Read the model definition and answer for the solid it produces. Units are mm, in the model's axes. A direction names the side the tool comes from. Coordinates: 2 decimals unless noted, no trailing zeros. Write each loop counter-clockwise with the first axis right and the second up, starting at its lowest first coordinate (ties: lowest second). Pieces come first, ordered by that corner, then holes.
1) The part is cut by section B-B (x = -1). Determine the outline of the cut face in (y, z), then the cut area to 3 significant figures.
2) The part is cut by section A-A (y = 0). Determine the outline of the cut face in (x, z).
3) The part is cut by section C-C (z = -6). Determine the outline of the cut face in (x, y).
4) Which of the six approach directions +Z, -Z, +X, -X, +Y, -Y give full straight-line access (tool end or side, diameter ignored) to faces 4 (the face through (-8, 0, 32.5)), 5 (the face through (8, 2.301, 31)), 6 (the face through (-0.218, 0.976, -9.535)), 7 (the face through (3, 0, -1)), 8 (the face through (-7.001, 0, 30.5))?
5) Each of these flat-tipped pins is pushed along its axis until it touches: pin 1 Ø0.6 at (x, z) = (7.5, 31.5) entering from +Y; pin 2 Ø6 at (x, z) = (3.5, 5) entering from -Y; pin 3 Ø0.6 at (x, z) = (-8, 32) entering from -Y. Where does it stop, or does it pass through?
6) Determine the mould class of faces 1 (the face through (8, 0, 32.5)), 2 (the face through (-0.2, 1.3, -7)), 3 (the face through (8.188, 0, 30.5)) for opening direction Z: +Z half, -Z half, draft (parallel to the pull), parting line (faces both ways), or undercut.
7) The part is cut by section D-D (y = -3.5). Determine the outline of the cut face in (x, z), then the cut area to 3 significant figures.
8) Find the intervals of material crossed by line 1 (Z direction, x = -3, y = -9.25); line 2 (Z direction, x = -2, y = 0.75); line 3 (Y direction, x = 0.5, z = 26), in increasing order.
from build123d import *

# Parameters (mm, degrees)
SKETCH1_R           = 11
BOSS_EXTRUDE1_DEPTH = 30
SKETCH2_R           = 3
BOSS_EXTRUDE2_DEPTH = 2
SKETCH3_R           = 2
BOSS_EXTRUDE3_DEPTH = 10
SKETCH4_W           = 1.187251635
SKETCH4_H           = 4.601713706
BOSS_EXTRUDE4_DEPTH = 3
SKETCH5_W           = 1.771317087
SKETCH5_H           = 3.201713706
CUT_EXTRUDE1_DEPTH  = 40.726440378
CUT_EXTRUDE2_DEPTH  = 5


with BuildPart() as part:
    # Sketch1 → Boss-Extrude1 (new body)
    with BuildSketch(Plane.XY):
        Circle(SKETCH1_R)
    extrude(amount=BOSS_EXTRUDE1_DEPTH)

    # Sketch2 → Boss-Extrude2 (add)
    with BuildSketch(Plane(origin=(0, 0, 0), x_dir=(-1, 0, 0), z_dir=(0, 0, -1))):
        Circle(SKETCH2_R)
    extrude(amount=BOSS_EXTRUDE2_DEPTH)

    # Sketch3 → Boss-Extrude3 (add)
    with BuildSketch(Plane(origin=(0, 0, -2), x_dir=(-1, 0, 0), z_dir=(0, 0, -1))):
        Circle(SKETCH3_R)
    extrude(amount=BOSS_EXTRUDE3_DEPTH)

    # Sketch4 → Boss-Extrude4 (add)
    with BuildSketch(Plane.XY.offset(30)):
        with Locations((-7.594653551, 0)):
            Rectangle(SKETCH4_W, SKETCH4_H)
        with Locations((7.594653551, 0)):
            Rectangle(SKETCH4_W, SKETCH4_H)
    extrude(amount=BOSS_EXTRUDE4_DEPTH)

    # Sketch5 → Cut-Extrude1 (cut, through all)
    with BuildSketch(Plane.ZY.offset(8.188279368)):
        with Locations((31.614341457, 0)):
            Rectangle(SKETCH5_W, SKETCH5_H)
    extrude(amount=-CUT_EXTRUDE1_DEPTH, mode=Mode.SUBTRACT)

    # Sketch6 → Cut-Extrude2 (cut)
    with BuildSketch(Plane(origin=(0, 0, -12), x_dir=(-1, 0, 0), z_dir=(0, 0, -1))):
        Polygon((-45.221186331, 12.264551338), (-1.439858088, 1.388095345), (1.922054875, 0.55290601), (45.703383118, -10.323549984), (67.456295106, 77.239106502), (-23.468274343, 99.827207824), align=None)
    extrude(amount=-CUT_EXTRUDE2_DEPTH, mode=Mode.SUBTRACT)


solid = part.part
Reported:
1. outline: (-10.95, 0) - (-2.83, 0) - (-2.83, -2) - (-1.73, -2) - (-1.73, -12) - (0.78, -12) - (0.78, -7) - (1.73, -7) - (1.73, -2) - (2.83, -2) - (2.83, 0) - (10.95, 0) - (10.95, 30) - (-10.95, 30) - close
1. area: 698 mm2
2. outline: (-11, 0) - (-3, 0) - (-3, -2) - (-2, -2) - (-2, -12) - (2, -12) - (2, -2) - (3, -2) - (3, 0) - (11, 0) - (11, 30) - (8.19, 30) - (8.19, 30.73) - (7, 30.73) - (7, 30) - (-7, 30) - (-7, 30.73) - (-8.19, 30.73) - (-8.19, 30) - (-11, 30) - close; (-8.19, 32.5) - (-7, 32.5) - (-7, 33) - (-8.19, 33) - close; (7, 32.5) - (8.19, 32.5) - (8.19, 33) - (7, 33) - close
3. outline: circle Ø4 at (0, 0)
4. face 4: +X, -X
4. face 5: +Z, +X, -X, +Y
4. face 6: -Z, -X, +Y
4. face 7: -Z
4. face 8: +Z, +Y, -Y
5. pin 1: stops at y = 2.3
5. pin 2: stops at y = -10.99
5. pin 3: stops at y = -2.3
6. face 1: undercut
6. face 2: -Z half
6. face 3: draft
7. outline: (-10.43, 0) - (10.43, 0) - (10.43, 30) - (-10.43, 30) - close
7. area: 626 mm2
8. line 1: z = 0 to 30
8. line 2: z = -2 to 30
8. line 3: y = -10.99 to 10.99
